Job drawing, mm, ordinate dimensions from the low corner. One solid piece. Give positions to 0.01 mm unless a question says otherwise; leave off trailing zeros. Order: outer loops, then holes, each group sorted by start corner. A loop starts at its lowest first (then second) coordinate and runs counter-clockwise, first axis right, second up.
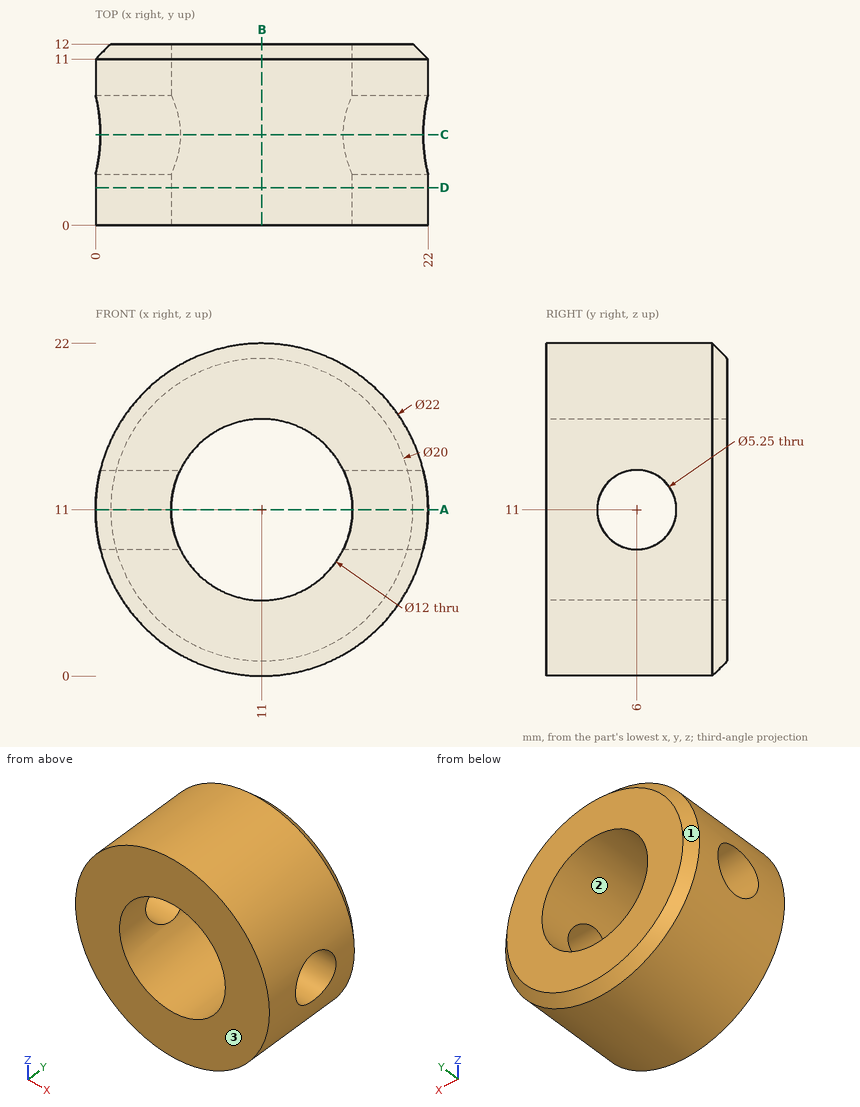
Item 1: Drop flat-ended pins along their axis: P1, Ø5, axis at x = 6, y = 5.5, coming from the +Z side; P2, Ø4, axis at y = 3, z = 18.5, coming from the +X side; P3, Ø10, axis at x = 15.5, z = 14.5, coming from the +Y side; P4, Ø2, axis at x = 2.5, y = 10.5, coming from the +Z side. Give the stop position or say it passes through.
Item 2: Pull direction Z, two halves, no side cores. Call the marked faces 1, 2 and 3: released by +Z, released by -Z, zero draft, split by the parting line, or undercut.
Item 3: Drill centre lines: probe 1 along Z at (x, y) = (11, 7.5); probe 2 along Z at (x, y) = (17.9, 6) (3 decimals); probe 3 along Y at (x, z) = (1.5, 10.5). Where is each one in solid material? Low to high.
Item 4: Band-saw the part on B-B on x = 11. List the corners of the cut face in (y, z).
Item 5: Band-saw the part on C-C on y = 6. List the corners of the cut face in (x, z) (3 decimals), plus the area to 3 significant figures.
Item 6: Band-saw the part on A-A on z = 11. List the corners of the cut face in (x, y) (3 decimals), plus the area to 3 significant figures.
Item 7: Band-saw the part on D-D on y = 2.5. List the corners of the cut face in (x, z).
Working result:
1. P1: stops at z = 21.71
1. P2: stops at x = 20.53
1. P3: stops at y = 12
1. P4: stops at z = 19.05
2. face 1: split by the parting line
2. face 2: undercut
2. face 3: zero draft
3. probe 1: z = 0 to 5, 17 to 22
3. probe 2: z = 2.433 to 8.375, 13.625 to 19.567
3. probe 3: y = 0 to 3.42, 8.58 to 12
4. outline: (0, 0) - (11, 0) - (12, 1) - (12, 5) - (0, 5) - close; (0, 17) - (12, 17) - (12, 21) - (11, 22) - (0, 22) - close
5. outline: (0.318, 8.375) arc R11 ccw to (21.682, 8.375) - (16.395, 8.375) arc R6 cw to (5.605, 8.375) - close; (0.318, 13.625) - (5.605, 13.625) arc R6 cw to (16.395, 13.625) - (21.682, 13.625) arc R11 ccw to start
5. area: 214 mm2
6. outline: (0, 0) - (5, 0) - (5, 3.375) - (0, 3.375) - close; (0, 8.625) - (5, 8.625) - (5, 12) - (1, 12) - (0, 11) - close; (17, 0) - (22, 0) - (22, 3.375) - (17, 3.375) - close; (17, 8.625) - (22, 8.625) - (22, 11) - (21, 12) - (17, 12) - close
6. area: 66.5 mm2
7. outline: circle Ø22 at (11, 11); hole circle Ø12 at (11, 11)
